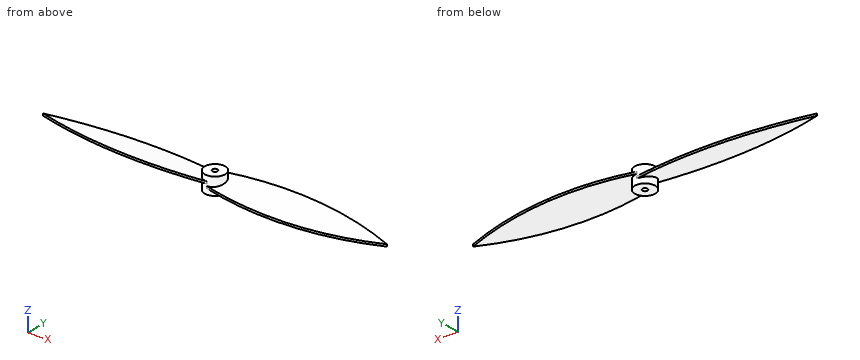
```python
from build123d import *

# Parameters (mm, degrees)
SKETCH1_R           = 6.000000000000002
SKETCH1_R_2         = 1.4999999999999918
BOSS_EXTRUDE1_DEPTH = 10
BOSS_EXTRUDE2_DEPTH = 125
CUT_EXTRUDE1_START  = -10.588348405
CUT_EXTRUDE1_DEPTH  = 11.17669681
CIRPATTERN1_COUNT   = 2


# Read off the part's stored shape, not the designer's step: Cut-Extrude1
with BuildPart() as part:
    # Sketch1 → Boss-Extrude1 (new body)
    with BuildSketch(Plane.XY):
        with Locations((0.1399887701091363, 164.8507075610879)):
            Circle(SKETCH1_R)
        with Locations((0.1399887701091363, 164.8507075610879)):
            Circle(SKETCH1_R_2, mode=Mode.SUBTRACT)
    extrude(amount=-BOSS_EXTRUDE1_DEPTH)

    # Sketch2 → Boss-Extrude2 (add)
    with BuildSketch(Plane(origin=(0, 0, 0), x_dir=(0, 0, -1), z_dir=(1, 0, 0))):
        Polygon((-0.5883484054145544, 189.73303788000499), (9.411651594585447, 139.73303788000499), (10.58834840541455, 139.9683772421708), (0.5883484054145496, 189.9683772421708), align=None)
    boss_extrude2 = extrude(amount=BOSS_EXTRUDE2_DEPTH)

    # Cut-Extrude1 outline → Cut-Extrude1 (cut)
    with BuildSketch(Plane.XY.offset(CUT_EXTRUDE1_START)):
        with BuildLine():
            Line((0, 170.850707561), (0.13998877, 170.850707561))
            ThreePointArc((0.13998877, 170.850707561), (50.466362146, 174.447589067), (100, 164.850707561))
            ThreePointArc((100, 164.850707561), (50.466362146, 155.253826055), (0.13998877, 158.850707561))
            Line((0.13998877, 158.850707561), (0, 158.850707561))
            Line((0, 158.850707561), (0, 131.123594735))
            Line((0, 131.123594735), (135.475544018, 131.123594735))
            Line((135.475544018, 131.123594735), (135.475544018, 197.042094646))
            Line((135.475544018, 197.042094646), (0, 197.042094646))
            Line((0, 197.042094646), (0, 170.850707561))
        make_face()
    cut_extrude1 = extrude(amount=CUT_EXTRUDE1_DEPTH, mode=Mode.SUBTRACT)

    # CirPattern1: Boss-Extrude2, Cut-Extrude1 ×2 about axis
    cirpattern1_axis = Axis((0.1399887701089445, 164.85070756108797, 0), (0, 0, 1))
    add([boss_extrude2.rotate(cirpattern1_axis, i * 360 / CIRPATTERN1_COUNT) for i in range(1, CIRPATTERN1_COUNT)])
    add([cut_extrude1.rotate(cirpattern1_axis, i * 360 / CIRPATTERN1_COUNT) for i in range(1, CIRPATTERN1_COUNT)], mode=Mode.SUBTRACT)


solid = part.part
```
Part model, mm, in its own coordinate system. Round coordinates to 2 decimals unless told otherwise and drop trailing zeros. Order: outer loops, then holes, each group sorted by start corner. A loop starts at its lowest first (then second) coordinate and runs counter-clockwise, first axis right, second up. Notation, with made-up numbers: M -7,17.25 L 3,17.25 A29 ccw 3,52.25 Z; hole C 46.5,-28.5 d3. An arc over 180 degrees is marked long. Answer in a Markdown table with one row per item. Add a question column.
Q1. Cut at C-C on x = -55. Give the cut face in (y, z).
Q2. Wall check: L1, parallel to Z at x = -65, y = 158.75; L2, parallel to Z at x = 59, y = 166.5; L3, parallel to Y at x = -1, z = -1.25. Give the ranges that are in metal, low to high. Write a range as from..to.
Q3. Pin check, flat tips, straight feed: pin 1 (5 mm diameter, centred on x = -2, z = -1, fed in from -Y); pin 2 (4 mm diameter, centred on y = 163, z = -6, fed in from -X); pin 3 (2 mm diameter, centred on x = -14, z = -7.5, fed in from +Y); pin 4 (1.8 mm diameter, centred on x = 0.14, y = 164.85, fed in from -Z). Stop position of each tip, or through.
Q4. Cut at A-A on y = 168.5. Give the cut face in (x, z).
Q5. Cut at B-B on x = 46. Give the cut face in (y, z), and give its area (3 significant figures).
Established:
| question | item | result |
|---|---|---|
| 1 | outline | M 155.6,-3.76 L 174.1,-7.46 L 174.1,-6.24 L 155.6,-2.54 Z |
| 2 | L1 | z = -4.39..-3.17 |
| 2 | L2 | z = -5.28..-4.06 |
| 2 | L3 | y = 158.96..163.88, 165.83..170.74 |
| 3 | pin 1 | stops at y = 158.15 |
| 3 | pin 2 | stops at x = -99.72 |
| 3 | pin 3 | stops at y = 173.34 |
| 3 | pin 4 | stops at z = -5.79 |
| 4 | outline | M -87.47,-6.34 L -4.62,-6.34 L -4.62,-10 L 4.9,-10 L 4.9,-4.88 L 87.75,-4.88 L 87.75,-3.66 L 4.9,-3.66 L 4.9,0 L -4.62,0 L -4.62,-5.12 L -87.47,-5.12 Z |
| 5 | outline | M 155.04,-7.57 L 174.66,-3.65 L 174.66,-2.43 L 155.04,-6.35 Z |
| 5 | area | 24.0 mm2 |
